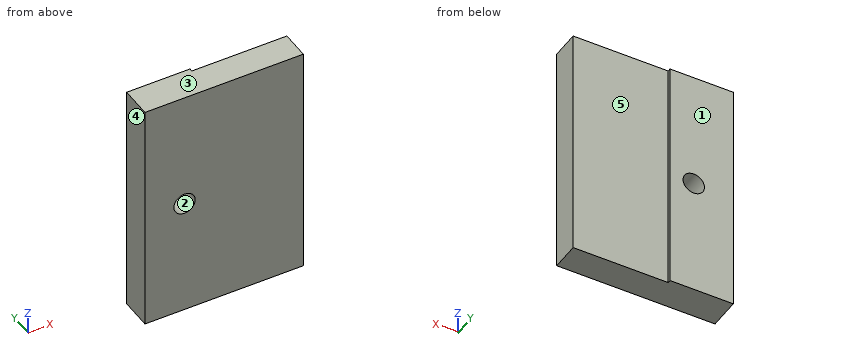
from build123d import *

# Parameters (mm, degrees)
F0_W     = 20
F0_H     = 30
F1_DEPTH = 4
F2_W     = 12
F2_H     = 30
F3_DEPTH = 0.4
F5_D     = 2.7


with BuildPart() as f1:
    # F0 (on Front) → F1 (new body)
    with BuildSketch(Plane.XZ):
        with Locations((10, 15)):
            Rectangle(F0_W, F0_H)
    extrude(amount=F1_DEPTH)

    # F2 (on Front) → F3 (cut)
    with BuildSketch(Plane.XZ):
        with Locations((14, 15)):
            Rectangle(F2_W, F2_H)
    extrude(amount=F3_DEPTH, mode=Mode.SUBTRACT)

    # F5 (through all)
    with Locations(Plane.XZ.offset(4)):
        with Locations((5, 15)):
            Hole(F5_D / 2)


solid = f1.part
Geometry check sheet. Reference: the model listing, model coordinates, mm. Face numbers are marked on the shaded views. A direction names the side the tool comes from. Give positions to 0.01 mm unless a question says otherwise; leave off trailing zeros. Loops run counter-clockwise (first coordinate to the right, second up) from the corner with the lowest first, then second, coordinate; pieces in that order, holes last. Notation, with made-up numbers: M 21,4 L 74,4 A24 ccw 74,31 Z; hole C 11,87.5 d4. An arc over 180 degrees is marked long. Answer as a JSON object with one key per item and string values. Group by question number.
Item 1: Material ranges on L1, parallel to Z at x = 5, y = -1.2; L2, parallel to Y at x = 17.5, z = 7; L3, parallel to X at y = -0.3, z = 2.5, recorded low to high.
Item 2: Sectioned sample at A-A on z = 15. Record the boundary of the cut face in (x, y), plus the area to 3 significant figures.
Item 3: Sectioned sample at D-D on x = 15.5. Record the boundary of the cut face in (y, z), plus the area to 3 significant figures.
Item 4: Sectioned sample at B-B on x = 5. Record the boundary of the cut face in (y, z).
Item 5: Sectioned sample at C-C on z = 19.75. Record the boundary of the cut face in (x, y), plus the area to 3 significant figures.
Item 6: Gauge pin test, flat ends, axial feed: pin 1 (9.5 mm diameter, centred on x = 13, z = 19, fed in from +Y); pin 2 (1.6 mm diameter, centred on x = 5, z = 15, fed in from +Y); pin 3 (1.5 mm diameter, centred on x = 3, y = -0.5, fed in from -Z). Record the tip position at first contact, or that the pin passes through.
Item 7: Access from +Z, -Z, +X, -X, +Y, -Y to the whole of each face (thin tool, end or side, straight path). Record for the marked faces 4 and 5.
Item 8: Mould release check, pull along Z, two halves, no side actions. Record for the marked faces 1, 2 and 3: pulls with the +Z half, pulls with the -Z half, needs draft (parallel to the pull), parting line crosses it, or undercut.
Findings below:
{
 "1": {"L1": "0 to 13.65, 16.35 to 30", "L2": "-4 to -0.4", "L3": "0 to 8"},
 "2": {"outline": "M 0,-4 L 3.65,-4 L 3.65,0 L 0,0 Z; M 6.35,-4 L 20,-4 L 20,-0.4 L 8,-0.4 L 8,0 L 6.35,0 Z", "area": "64.4 mm2"},
 "3": {"outline": "M -4,0 L -0.4,0 L -0.4,30 L -4,30 Z", "area": "108 mm2"},
 "4": {"outline": "M -4,0 L 0,0 L 0,13.65 L -4,13.65 Z; M -4,16.35 L 0,16.35 L 0,30 L -4,30 Z"},
 "5": {"outline": "M 0,-4 L 20,-4 L 20,-0.4 L 8,-0.4 L 8,0 L 0,0 Z", "area": "75.2 mm2"},
 "6": {"pin 1": "y = -0.4", "pin 2": "through", "pin 3": "z = 0"},
 "7": {"face 4": "+Z, -Z, -X, +Y, -Y", "face 5": "+Z, -Z, +X, +Y"},
 "8": {"face 1": "needs draft", "face 2": "undercut", "face 3": "pulls with the +Z half"}
}
